from build123d import *

# Parameters (mm, degrees)
BOSS_EXTRUDE1_DEPTH = 2
SKETCH4_R           = 1.5
CUT_EXTRUDE1_DEPTH  = 8
SCALE1_SCALE        = 2


with BuildPart() as part:
    # Sketch2 → Revolve1 (revolve)
    with BuildSketch(Plane(origin=(0, 0, 0), x_dir=(0, 0, -1), z_dir=(1, 0, 0))):
        Polygon((0, 0), (-5, 0), (-5, 3), (-1.5, 3), (-1.5, 4), (-5, 4), (-5, 5), (-1, 5), (-1, 4), (1, 4), (1, 5), (5, 5), (5, 4), (1.5, 4), (1.5, 0), align=None)
    revolve(axis=Axis((0, 0, 7.547271319), (0, 0, -1)))

    # Sketch3 → Boss-Extrude1 (add)
    with BuildSketch(Plane(origin=(0, 0, -1.5), x_dir=(-1, 0, 0), z_dir=(0, 0, -1))):
        with BuildLine():
            Line((0.5, 1.936491673), (0.5, 3.968626967))
            ThreePointArc((0.5, 3.968626967), (0, 4), (-0.5, 3.968626967))
            Line((-0.5, 3.968626967), (-0.5, 1.936491673))
            ThreePointArc((-0.5, 1.936491673), (-1.414213562, 1.414213562), (-1.936491673, 0.5))
            Line((-1.936491673, 0.5), (-3.968626967, 0.5))
            ThreePointArc((-3.968626967, 0.5), (-4, 0), (-3.968626967, -0.5))
            Line((-3.968626967, -0.5), (-1.936491673, -0.5))
            ThreePointArc((-1.936491673, -0.5), (-1.414213562, -1.414213562), (-0.5, -1.936491673))
            Line((-0.5, -1.936491673), (-0.5, -3.968626967))
            ThreePointArc((-0.5, -3.968626967), (0, -4), (0.5, -3.968626967))
            Line((0.5, -3.968626967), (0.5, -1.936491673))
            ThreePointArc((0.5, -1.936491673), (1.414213562, -1.414213562), (1.936491673, -0.5))
            Line((1.936491673, -0.5), (3.968626967, -0.5))
            ThreePointArc((3.968626967, -0.5), (4, 0), (3.968626967, 0.5))
            Line((3.968626967, 0.5), (1.936491673, 0.5))
            ThreePointArc((1.936491673, 0.5), (1.414213562, 1.414213562), (0.5, 1.936491673))
        make_face()
    extrude(amount=BOSS_EXTRUDE1_DEPTH)

    # Sketch4 → Cut-Extrude1 (cut)
    with BuildSketch(Plane.XY.offset(5)):
        Circle(SKETCH4_R)
    extrude(amount=-CUT_EXTRUDE1_DEPTH, mode=Mode.SUBTRACT)


with BuildPart() as part_1:
    # Scale1: scaled about (0, 0, 0.351761007)
    add(part.part.scale(SCALE1_SCALE).moved(Location((0, 0, -0.351761007))))


solid = part_1.part
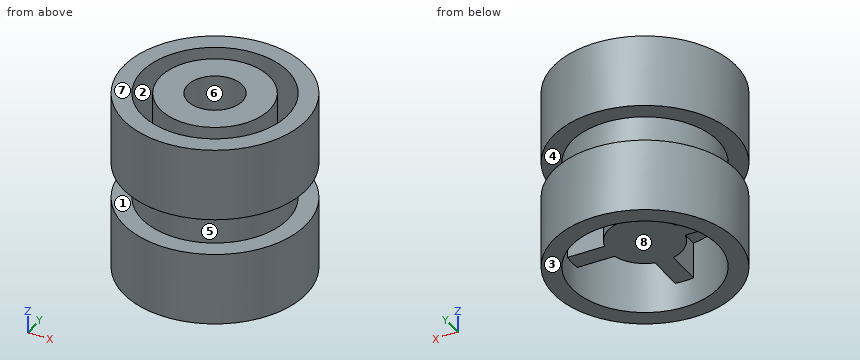
Could you check a few things on this model? Use its own coordinates, in mm. Face numbers are marked on the shaded views. A direction names the side the tool comes from. Give positions to 0.01 mm unless a question says otherwise; leave off trailing zeros. Order: outer loops, then holes, each group sorted by start corner. A loop starts at its lowest first (then second) coordinate and runs counter-clockwise, first axis right, second up. Notation, with made-up numbers: (-40, 43) - (-21, 43) arc R7 ccw to (-21, 48) - close; hole circle Ø7 at (48, -12). An arc over 180 degrees is marked (long way). One line per question, with ' | ' between items. Start each with the question number.
Item 1: I need wall thicknesses on probe 1 along X at (y, z) = (0.25, 4.25); probe 2 along X at (y, z) = (0, -8.5); probe 3 along X at (y, z) = (-2.75, 5.25). Which ranges of each line are inside material? Lowest first, please. Write a range as [from, to].
Item 2: I want a section at A-A on z = -7. Write out the boundary of the cut face in (x, y), then the cut area to 3 significant figures.
Item 3: Thinking about a two-plate mould opening in Z: for the marked faces 1, 2, 3 and 4, which applies, pulls with the +Z half, pulls with the -Z half, needs draft (parallel to the pull), parting line crosses it, or undercut?
Item 4: I want a section at B-B on x = 0. Write out the boundary of the cut face in (y, z).
Item 5: For the marked faces 5, 6, 7 and 8, which set-ups out of +Z, -Z, +X, -X, +Y, -Y let a thin tool reach every point of the face, with its end or its side?
Item 6: I want a section at C-C on z = 4.75. Write out the boundary of the cut face in (x, y), then the cut area to 3 significant figures.
Item 7: I'm going to push flat-ended pins straight in: pin 1 Ø1.5 at (x, y) = (-3.5, 5) entering from -Z; pin 2 Ø1.5 at (x, z) = (-0.5, 0.5) entering from -Y; pin 3 Ø3 at (x, z) = (5.5, -6) entering from +Y. Where does each tip first touch, or does it pass through?
Verdict:
1) probe 1: [-10, -8], [-5.99, -2.99], [2.99, 5.99], [8, 10] | probe 2: [-10, -8], [8, 10] | probe 3: [-9.61, -7.51], [-5.33, -1.2], [1.2, 5.33], [7.51, 9.61]
2) outline: circle Ø20 at (0, 0); hole (-7.94, -1) arc R8 ccw to (-1, -7.94) - (-1, -3.87) arc R4 cw to (-3.87, -1) - close; hole (-7.94, 1) - (-3.87, 1) arc R4 cw to (-1, 3.87) - (-1, 7.94) arc R8 ccw to start; hole (1, -7.94) arc R8 ccw to (7.94, -1) - (3.87, -1) arc R4 cw to (1, -3.87) - close; hole (1, 3.87) arc R4 cw to (3.87, 1) - (7.94, 1) arc R8 ccw to (1, 7.94) - close | area: 196 mm^2
3) face 1: undercut | face 2: needs draft | face 3: pulls with the -Z half | face 4: undercut
4) outline: (-10, -10.35) - (-8, -10.35) - (-8, -7.35) - (8, -7.35) - (8, -10.35) - (10, -10.35) - (10, -2.35) - (8, -2.35) - (8, 1.65) - (10, 1.65) - (10, 9.65) - (8, 9.65) - (8, 2.65) - (6, 2.65) - (6, 9.65) - (3, 9.65) - (3, -6.35) - (-3, -6.35) - (-3, 9.65) - (-6, 9.65) - (-6, 2.65) - (-8, 2.65) - (-8, 9.65) - (-10, 9.65) - (-10, 1.65) - (-8, 1.65) - (-8, -2.35) - (-10, -2.35) - close
5) face 5: none | face 6: +Z | face 7: +Z, +X, -X, +Y, -Y | face 8: -Z
6) outline: circle Ø20 at (0, 0); circle Ø12 at (0, 0); hole circle Ø16 at (0, 0); hole circle Ø6 at (0, 0) | area: 198 mm^2
7) pin 1: z = -3.35 | pin 2: y = -8 | pin 3: y = 9.17
